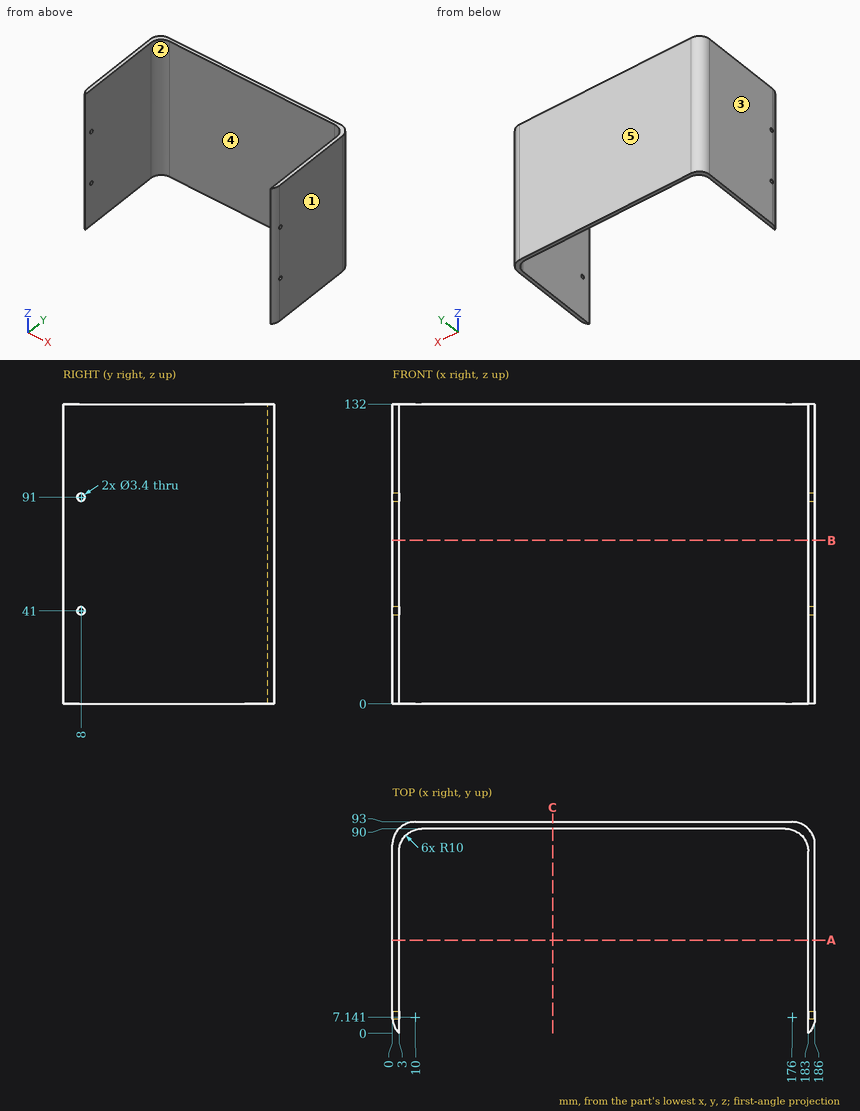
Geometry: see drawing. Coordinates: mm, zero at the bounding-box minimum. A direction names the side the tool comes from. Round coordinates to 2 decimals unless told otherwise and drop trailing zeros. Write each loop counter-clockwise with the first axis right and the second up, starting at its lowest first coordinate (ties: lowest second). Pieces come first, ordered by that corner, then holes. Notation, with made-up numbers: M -20.75,85 L 33.25,85 A26 ccw 33.25,111 Z; hole C -20,12 d2. An arc over 180 degrees is marked long. Answer in a Markdown table with one row per item. Add a question column.
(1) Reachability of the marked faces 1 and 2 from +Z, -Z, +X, -X, +Y, -Y: full face, straight path, thin tool, end or side. Return the list, or none.
(2) Cut plane C-C, the plane x = 70.5. Return the cut outline in (y, z).
(3) Draft query along X for the marked faces 3, 4 and 5. Return one class per face: pulls with the +X half, pulls with the -X half, needs draft (parallel to the pull), parting line crosses it, or undercut.
(4) Cut plane A-A, the plane y = 41. Return the cut outline in (x, z).
(5) Cut plane B-B, the plane z = 72. Return the cut outline in (x, y).
(6) Contact query for flat-ended pins moving along their axis: pin 1 (8 mm diameter, centred on x = 163, z = 61.5, fed in from -Y); pin 2 (3 mm diameter, centred on y = 8, z = 41, fed in from -X). Output: stop coordinate, or through.
(7) Ray query, L1, parallel to X at y = 75, z = 31.5; L2, parallel to Y at x = 100, z = 88.5; L3, parallel to X at y = 87, z = 14 (1 decimal). Return the intervals inside material, ascending.
Established:
| question | item | result |
|---|---|---|
| 1 | face 1 | +Z, -Z, +X, +Y, -Y |
| 1 | face 2 | +Z, -Z, -Y |
| 2 | outline | M 90,0 L 93,0 L 93,132 L 90,132 Z |
| 3 | face 3 | pulls with the -X half |
| 3 | face 4 | undercut |
| 3 | face 5 | needs draft |
| 4 | outline | M 0,0 L 3,0 L 3,132 L 0,132 Z; M 183,0 L 186,0 L 186,132 L 183,132 Z |
| 5 | outline | M 0,7.14 A10 ccw 3,0 L 3,80 A10 cw 13,90 L 173,90 A10 cw 183,80 L 183,0 A10 ccw 186,7.14 L 186,83 A10 ccw 176,93 L 10,93 A10 ccw 0,83 Z |
| 6 | pin 1 | y = 90 |
| 6 | pin 2 | through |
| 7 | L1 | 0 to 3, 183 to 186 |
| 7 | L2 | 90 to 93 |
| 7 | L3 | 0.8 to 5.9, 180.1 to 185.2 |
